Check sheet for the modelled part. Datum: model origin and axes. Units: mm. A direction names the side the tool comes from. Give positions to 0.01 mm unless a question says otherwise; leave off trailing zeros. Write each loop counter-clockwise with the first axis right and the second up, starting at its lowest first coordinate (ties: lowest second). Pieces come first, ordered by that corner, then holes. Notation, with made-up numbers: (40, -22) - (69, -22) arc R9 ccw to (69, -10) - close; hole circle Ø7 at (18, 61.25). An arc over 180 degrees is marked (long way). Return JSON: item names as keys, results as strings. Group by question number.
```python
from build123d import *

# Parameters (mm, degrees)
SKETCH1_R                    = 6.349999999
SKETCH1_R_2                  = 3
BOSS_EXTRUDE1_DEPTH          = 4.7625
FILLET1_R                    = 5.08
F_3_0_3_DIAMETER_HOLE1_D     = 3
F_3_0_3_DIAMETER_HOLE1_DEPTH = 25.4
F_3_0_3_DIAMETER_HOLE1_TIP   = 0.901290929


with BuildPart() as part:
    # Sketch1 → Boss-Extrude1 (new body)
    with BuildSketch(Plane.XY):
        Polygon((528.484361343, 22.816913392), (448.484361343, 22.816913392), (448.484361343, -17.183086608), (488.484361343, -17.183086608), (488.484361343, -34.703086608), (528.484361343, -34.703086608), align=None)
        with Locations(Location((507.054361343, -25.943086608, 0), (0, 0, 180))):
            Circle(SKETCH1_R, mode=Mode.SUBTRACT)
        with Locations(Location((464.484361343, 2.816913392, 0), (0, 0, 180))):
            Circle(SKETCH1_R_2, mode=Mode.SUBTRACT)
        with Locations(Location((519.484361343, 2.816913392, 0), (0, 0, 180))):
            Circle(SKETCH1_R_2, mode=Mode.SUBTRACT)
        with BuildLine():
            Line((490.984361343, 6.816913392), (505.984361343, 6.816913392))
            ThreePointArc((505.984361343, 6.816913392), (509.984361343, 2.816913392), (505.984361343, -1.183086608))
            Line((505.984361343, -1.183086608), (490.984361343, -1.183086608))
            ThreePointArc((490.984361343, -1.183086608), (486.984361343, 2.816913392), (490.984361343, 6.816913392))
        make_face(mode=Mode.SUBTRACT)
    extrude(amount=BOSS_EXTRUDE1_DEPTH)

    # Fillet1
    fillet1_edges = [part.edges().sort_by_distance(p)[0] for p in [
        (528.484361343, -34.703086608, 2.38125),
        (488.484361343, -34.703086608, 2.38125),
        (488.484361343, -17.183086608, 2.38125),
        (448.484361343, -17.183086608, 2.38125),
        (448.484361343, 22.816913392, 2.38125),
        (528.484361343, 22.816913392, 2.38125),
    ]]
    fillet(fillet1_edges, radius=FILLET1_R)

    # Ø3.0 (3) Diameter Hole1
    with Locations(Plane(origin=(0, 0, 0), x_dir=(-1, 0, 0), z_dir=(0, 0, -1))):
        with Locations((-497.524361343, -25.943086608), (-516.584361343, -25.943086608)):
            Hole(F_3_0_3_DIAMETER_HOLE1_D / 2, depth=F_3_0_3_DIAMETER_HOLE1_DEPTH)
            with Locations((0, 0, -(F_3_0_3_DIAMETER_HOLE1_DEPTH + F_3_0_3_DIAMETER_HOLE1_TIP / 2))):  # 118° drill point
                Cone(0, F_3_0_3_DIAMETER_HOLE1_D / 2, F_3_0_3_DIAMETER_HOLE1_TIP, mode=Mode.SUBTRACT)


solid = part.part
```
Item 1: Mould release check, pull along X, two halves, no side actions. Record for faces 1 (the face through (488, -6, 4.762)), 2 (the face through (486.957, -18.632, 2.415)), 3 (the face through (526.957, 21.368, 2.415)), 4 (the face through (498, 6.817, 2)): +X half, -X half, draft (parallel to the pull), parting line (faces both ways), or undercut.
Item 2: Section check B-B on z = 2.4. Record the cut outline in (x, y).
Item 3: Access from +Z, -Z, +X, -X, +Y, -Y to the whole of each face (thin tool, end or side, straight path). Record for faces 5 (the face through (468, -17.183, 2)), 6 (the face through (488, -6, 0)), 7 (the face through (499, -1.183, 2)).
Item 4: Section check A-A on x = 504. Record the cut outline in (y, z), plus the area to 3 significant figures.
Item 5: Material ranges on line 1 along Y through (x, z) = (505, 2.25); line 2 along X through (y, z) = (1, 3.6); line 3 along Y through (x, z) = (466.5, 0.95), recorded low to high. Write a range as from..to.
Item 6: Section check C-C on x = 472.5. Record the cut outline in (y, z).
Item 7: Section check D-D on x = 485. Record the cut outline in (y, z), plus the area to 3 significant figures.
Item 8: Depth check by flat-ended pin: pin 1 (7 mm diameter, centred on x = 464.48, y = 2.82, fed in from +Z); pin 2 (1.4 mm diameter, centred on x = 463, z = 2, fed in from -Y); pin 3 (11.5 mm diameter, centred on x = 507.05, y = -25.94, fed in from -Z). Enter the tip coordinate at first touch or a pass-through.
Reply:
{
 "1": {"face 1": "draft", "face 2": "-X half", "face 3": "+X half", "face 4": "undercut"},
 "2": {"outline": "(448.48, -12.1) arc R5.08 ccw to (453.56, -17.18) - (483.4, -17.18) arc R5.08 cw to (488.48, -22.26) - (488.48, -29.62) arc R5.08 ccw to (493.56, -34.7) - (523.4, -34.7) arc R5.08 ccw to (528.48, -29.62) - (528.48, 17.74) arc R5.08 ccw to (523.4, 22.82) - (453.56, 22.82) arc R5.08 ccw to (448.48, 17.74) - close; hole circle Ø6 at (464.48, 2.82); hole (490.98, -1.18) - (505.98, -1.18) arc R4 ccw to (505.98, 6.82) - (490.98, 6.82) arc R4 ccw to start; hole circle Ø3 at (497.52, -25.94); hole circle Ø12.7 at (507.05, -25.94); hole circle Ø3 at (516.58, -25.94); hole circle Ø6 at (519.48, 2.82)"},
 "3": {"face 5": "+Z, -Z, -X, -Y", "face 6": "-Z, +X, -X, +Y, -Y", "face 7": "+Z, -Z"},
 "4": {"outline": "(-34.7, 0) - (-31.51, 0) - (-31.51, 4.76) - (-34.7, 4.76) - close; (-20.38, 0) - (-1.18, 0) - (-1.18, 4.76) - (-20.38, 4.76) - close; (6.82, 0) - (22.82, 0) - (22.82, 4.76) - (6.82, 4.76) - close", "area": "183 mm²"},
 "5": {"line 1": "-34.7..-31.95, -19.93..-1.18, 6.82..22.82", "line 2": "448.48..462.1, 466.87..487.42, 509.55..517.1, 521.87..528.48", "line 3": "-17.18..0.59, 5.04..22.82"},
 "6": {"outline": "(-17.18, 0) - (22.82, 0) - (22.82, 4.76) - (-17.18, 4.76) - close"},
 "7": {"outline": "(-17.44, 0) - (22.82, 0) - (22.82, 4.76) - (-17.44, 4.76) - close", "area": "192 mm²"},
 "8": {"pin 1": "z = 4.76", "pin 2": "y = -17.18", "pin 3": "through"}
}
